The model under review builds one solid part; all positions refer to its coordinate system, in mm. A direction names the side the tool comes from. Round coordinates to 2 decimals unless told otherwise and drop trailing zeros. Write each loop counter-clockwise with the first axis right and the second up, starting at its lowest first coordinate (ties: lowest second). Pieces come first, ordered by that corner, then holes. Notation, with made-up numbers: M 81,-26 L 92,-26 A20 ccw 92,-14 Z; hole C 85,33.5 d3. An arc over 180 degrees is marked long. Write item = value, one per line. Start each with the question number.
Item 1: The part is to be moulded in two halves that separate along Z. For faces 4 (the cylindrical face through (3.51, 5.83, 9.64)), 5 (the cylindrical face through (1.972, -10.648, 13.887)), 6 (the flat face through (0, -4, -4)), say which applies: +Z half, -Z half, draft (parallel to the pull), parting line (faces both ways), or undercut.
Item 2: Take a section at C-C, the plane z = -7.5. Give the boundary of the cut face in (x, y), plus the area to 3 significant figures.
Item 3: Tool access review of faces 1 (the cylindrical face through (3.507, -11.265, 0.228)), 2 (the flat face through (3.01, 10.55, -2.22)), 3 (the cylindrical face through (1.48, 10.07, -0.65)): name each direction out of +Z, -Z, +X, -X, +Y, -Y from which nothing blocks a thin tool from reaching the whole face with its end or side.
Item 4: Take a section at A-A, the plane y = 0. Give the boundary of the cut face in (x, z), plus the area to 3 significant figures.
Item 5: To check wall thickness, follow line 1 along Y through (x, z) = (1.55, 0); line 2 along Y through (x, z) = (1, -13); line 3 along Z through (x, y) = (2.75, 5.5). State the ranges of each line that lie inside material, in increasing order.
Item 6: Take a section at D-D, the plane y = -9. Give the boundary of the cut face in (x, z), plus the area to 3 significant figures.
Item 7: Take a section at B-B, the plane y = 5.5. Give the boundary of the cut face in (x, z), plus the area to 3 significant figures.
Item 8: For pin 1 Ø5.5 at (y, z) = (-13, 0) entering from -X, flat-tipped, find the tip position at first contact; note if it passes through.
from build123d import *

# Parameters (mm, degrees)
SKETCH1_R           = 17.5
SKETCH1_R_2         = 4.75
BOSS_EXTRUDE1_DEPTH = 4
CUT_EXTRUDE1_DEPTH  = 2
SKETCH3_R           = 1.75
CUT_EXTRUDE2_DEPTH  = 26.069902273
SKETCH4_R           = 3
CUT_EXTRUDE3_DEPTH  = 3


with BuildPart() as part:
    # Sketch1 → Boss-Extrude1 (new body)
    with BuildSketch(Plane(origin=(0, 0, 0), x_dir=(0, 0, -1), z_dir=(1, 0, 0))):
        Circle(SKETCH1_R)
        Circle(SKETCH1_R_2, mode=Mode.SUBTRACT)
    extrude(amount=BOSS_EXTRUDE1_DEPTH)

    # Sketch2 → Cut-Extrude1 (cut)
    with BuildSketch(Plane(origin=(4, 0, 0), x_dir=(0, 0, -1), z_dir=(1, 0, 0))):
        with BuildLine():
            Line((13.567828444, -2.639615665), (7.013907066, -4.049481133))
            Line((7.013907066, -4.049481133), (9.069888444, -10.430276274))
            ThreePointArc((9.069888444, -10.430276274), (7.85, -13.596598839), (4.49794, -13.069891939))
            Line((4.49794, -13.069891939), (0, -8.098962266))
            Line((0, -8.098962266), (-4.49794, -13.069891939))
            ThreePointArc((-4.49794, -13.069891939), (-7.85, -13.596598839), (-9.069888444, -10.430276274))
            Line((-9.069888444, -10.430276274), (-7.013907066, -4.049481133))
            Line((-7.013907066, -4.049481133), (-13.567828444, -2.639615665))
            ThreePointArc((-13.567828444, -2.639615665), (-15.7, 0), (-13.567828444, 2.639615665))
            Line((-13.567828444, 2.639615665), (-7.013907066, 4.049481133))
            Line((-7.013907066, 4.049481133), (-9.069888444, 10.430276274))
            ThreePointArc((-9.069888444, 10.430276274), (-7.85, 13.596598839), (-4.49794, 13.069891939))
            Line((-4.49794, 13.069891939), (0, 8.098962266))
            Line((0, 8.098962266), (4.49794, 13.069891939))
            ThreePointArc((4.49794, 13.069891939), (7.85, 13.596598839), (9.069888444, 10.430276274))
            Line((9.069888444, 10.430276274), (7.013907066, 4.049481133))
            Line((7.013907066, 4.049481133), (13.567828444, 2.639615665))
            ThreePointArc((13.567828444, 2.639615665), (15.7, 0), (13.567828444, -2.639615665))
        make_face()
    extrude(amount=-CUT_EXTRUDE1_DEPTH, mode=Mode.SUBTRACT)

    # Sketch3 → Cut-Extrude2 (cut, through all)
    with BuildSketch(Plane(origin=(4, 0, 0), x_dir=(0, 0, -1), z_dir=(1, 0, 0))):
        with Locations((0, 13)):
            Circle(SKETCH3_R)
        with Locations((11.258330249, 6.5)):
            Circle(SKETCH3_R)
        with Locations((11.258330249, -6.5)):
            Circle(SKETCH3_R)
        with Locations((0, -13)):
            Circle(SKETCH3_R)
        with Locations((-11.258330249, -6.5)):
            Circle(SKETCH3_R)
        with Locations((-11.258330249, 6.5)):
            Circle(SKETCH3_R)
    extrude(amount=-CUT_EXTRUDE2_DEPTH, mode=Mode.SUBTRACT)

    # Sketch4 → Cut-Extrude3 (cut)
    with BuildSketch(Plane.ZY):
        with Locations((-11.258330249, 6.5)):
            Circle(SKETCH4_R)
        with Locations((0, 13)):
            Circle(SKETCH4_R)
        with Locations((11.258330249, 6.5)):
            Circle(SKETCH4_R)
        with Locations((11.258330249, -6.5)):
            Circle(SKETCH4_R)
        with Locations((0, -13)):
            Circle(SKETCH4_R)
        with Locations((-11.258330249, -6.5)):
            Circle(SKETCH4_R)
    extrude(amount=-CUT_EXTRUDE3_DEPTH, mode=Mode.SUBTRACT)


solid = part.part
Response values:
q1.face_4 = undercut
q1.face_5 = parting line
q1.face_6 = draft
q2.outline = M 0,-15.81 L 4,-15.81 L 4,-13.77 L 2,-13.77 L 2,-5.56 L 4,-5.56 L 4,-3.94 L 2,-3.94 L 2,3.94 L 4,3.94 L 4,5.56 L 2,5.56 L 2,13.77 L 4,13.77 L 4,15.81 L 0,15.81 Z
q2.area = 77.9 mm2
q3.face_1 = +X, -X
q3.face_2 = +X
q3.face_3 = -X
q4.outline = M 0,-17.5 L 4,-17.5 L 4,-15.7 L 2,-15.7 L 2,-4.75 L 0,-4.75 Z; M 0,4.75 L 2,4.75 L 2,15.7 L 4,15.7 L 4,17.5 L 0,17.5 Z
q4.area = 58.2 mm2
q5.line_1 = -17.5 to -16, -10 to -4.75, 4.75 to 10, 16 to 17.5
q5.line_2 = -11.72 to -8.94, -4.06 to 4.06, 8.94 to 11.72
q5.line_3 = -16.61 to -14.09, -8.43 to -7.48, 7.48 to 8.43, 14.09 to 16.61
q6.outline = M 0,-15.01 L 4,-15.01 L 4,-8.61 L 2,-8.61 L 2,-0.82 L 4,-0.82 L 4,0.82 L 2,0.82 L 2,8.61 L 4,8.61 L 4,15.01 L 0,15.01 L 0,12.92 L 3,12.92 L 3,9.6 L 0,9.6 L 0,-9.6 L 3,-9.6 L 3,-12.92 L 0,-12.92 Z
q6.area = 69.0 mm2
q7.outline = M 0,-16.61 L 4,-16.61 L 4,-12.69 L 3,-12.69 L 3,-14.09 L 0,-14.09 Z; M 0,-8.43 L 3,-8.43 L 3,-9.82 L 4,-9.82 L 4,-7.48 L 2,-7.48 L 2,7.48 L 4,7.48 L 4,9.82 L 3,9.82 L 3,8.43 L 0,8.43 Z; M 0,14.09 L 3,14.09 L 3,12.69 L 4,12.69 L 4,16.61 L 0,16.61 Z
q7.area = 63.3 mm2
q8.pin_1 = 3
